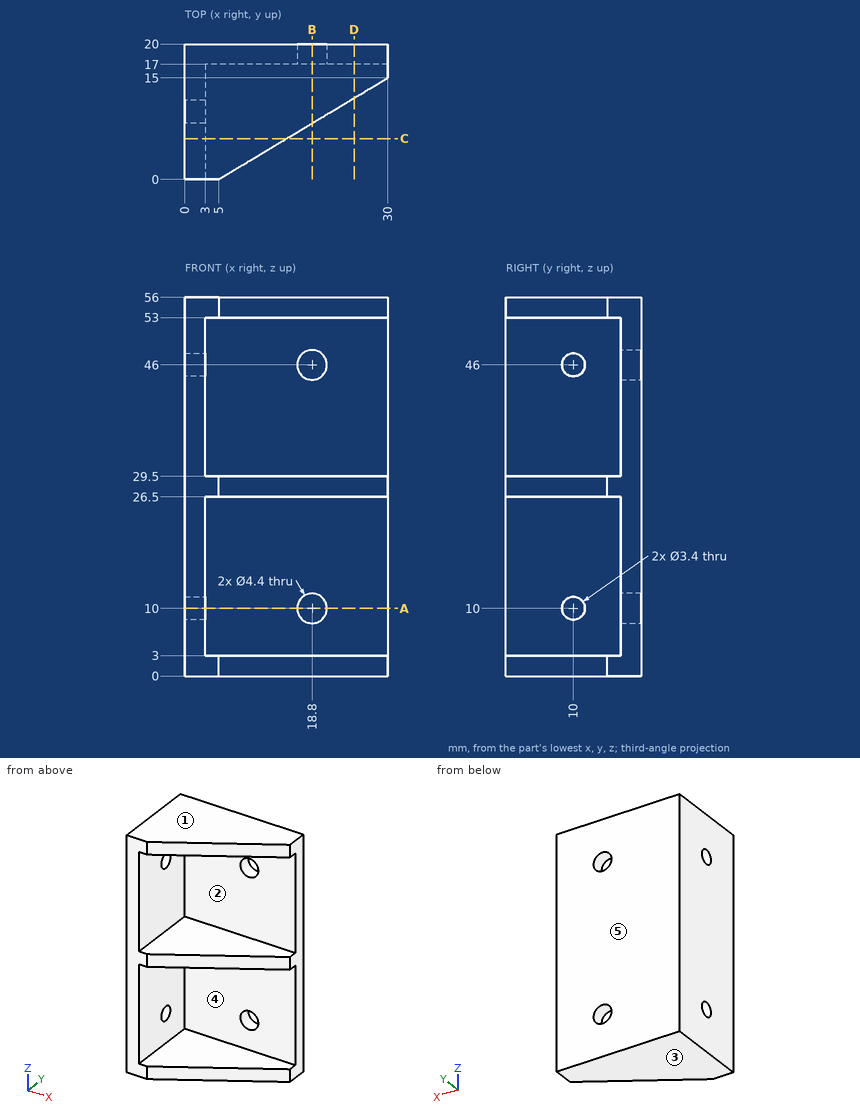
Could you check a few things on this drawing? It's one solid part, dimensions in mm from its lowest x, y, z. A direction names the side the tool comes from. Coordinates: 2 decimals unless noted, no trailing zeros. Order: outer loops, then holes, each group sorted by start corner. A loop starts at its lowest first (then second) coordinate and runs counter-clockwise, first axis right, second up. Notation, with made-up numbers: (49, 89) - (56, 89) arc R19 ccw to (56, 110) - close; hole circle Ø9 at (64, 69). An arc over 180 degrees is marked (long way). One line per question, with ' | ' between items. Start each with the question number.
1. Please list where these lines run through material, in increasing order: line 1 along Z through (x, y) = (4.5, 7.5); line 2 along Y through (x, z) = (0.75, 10); line 3 along Z through (x, y) = (18.75, 18.75). Write a range as [from, to].
2. If we section it at D-D (x = 25): Write out the boundary of the cut face in (y, z).
3. If we section it at B-B (x = 18.8): Write out the boundary of the cut face in (y, z).
4. If we section it at A-A (z = 10): Write out the boundary of the cut face in (x, y).
5. If we section it at C-C (y = 6): Write out the boundary of the cut face in (x, z).
6. I'm going to push flat-ended pins straight in: pin 1 Ø5 at (y, z) = (12, 20) entering from +X; pin 2 Ø7 at (x, z) = (14, 13.5) entering from -Y. Where does each tip first touch, or does it pass through?
7. Which directions (+Z, -Z, +X, -X, +Y, -Y) give clear straight access to the entire face, cutting with the end or side of a thin tool? Please do the marked faces 4 and 5.
8. If we mould it in two halves opening along Z, with no side actions, what happens to the marked faces 1, 2 and 3? For each: released by +Z, released by -Z, zero draft, split by the parting line, or undercut.
Model answer:
1) line 1: z = [0, 3], [26.5, 29.5], [53, 56] | line 2: y = [0, 8.3], [11.7, 20] | line 3: z = [0, 7.8], [12.2, 43.8], [48.2, 56]
2) outline: (12, 0) - (20, 0) - (20, 56) - (12, 56) - (12, 53) - (17, 53) - (17, 29.5) - (12, 29.5) - (12, 26.5) - (17, 26.5) - (17, 3) - (12, 3) - close
3) outline: (8.28, 0) - (20, 0) - (20, 7.8) - (17, 7.8) - (17, 3) - (8.28, 3) - close; (8.28, 26.5) - (17, 26.5) - (17, 12.2) - (20, 12.2) - (20, 43.8) - (17, 43.8) - (17, 29.5) - (8.28, 29.5) - close; (8.28, 53) - (17, 53) - (17, 48.2) - (20, 48.2) - (20, 56) - (8.28, 56) - close
4) outline: (0, 0) - (3, 0) - (3, 8.3) - (0, 8.3) - close; (0, 11.7) - (3, 11.7) - (3, 17) - (16.6, 17) - (16.6, 20) - (0, 20) - close; (21, 17) - (30, 17) - (30, 20) - (21, 20) - close
5) outline: (0, 0) - (15, 0) - (15, 3) - (3, 3) - (3, 26.5) - (15, 26.5) - (15, 29.5) - (3, 29.5) - (3, 53) - (15, 53) - (15, 56) - (0, 56) - close
6) pin 1: stops at x = 3 | pin 2: stops at y = 17
7) face 4: +X, -Y | face 5: +Z, -Z, +X, -X, +Y
8) face 1: released by +Z | face 2: undercut | face 3: released by -Z
